Design review of the part built by this model. Coordinates are the model's own, in mm. A direction names the side the tool comes from. Coordinates: 2 decimals unless noted, no trailing zeros. Order: outer loops, then holes, each group sorted by start corner. A loop starts at its lowest first (then second) coordinate and runs counter-clockwise, first axis right, second up. Notation, with made-up numbers: M -34,6.25 L 15,6.25 A9 ccw 15,13.25 Z; hole C 17,-21 d9. An arc over 180 degrees is marked long. Answer in a Markdown table with one row per item.
Autodesk Inventor part; units mm, degrees
ref_plane "YZ Plane" through (0, 0, 0) normal (1, 0, 0) x (0, 1, 0)
ref_plane "XZ Plane" through (0, 0, 0) normal (0, 1, 0) x (-1, 0, 0)
ref_plane "XY Plane" through (0, 0, 0) normal (0, 0, 1) x (1, 0, 0)
sketch "スケッチ1" plane through (0, 0, 0) normal (0, 0, 1) x (1, 0, 0)
  line L0 (0, 0) -> (24.7487, 24.7487) construction
  line L1 (0, 0) -> (8.6903, 0) construction
  circle A0 centre (7.0711, 7.0711) radius 1.75
  circle A1 centre (12.0208, 12.0208) radius 1.75
  circle A2 centre (24.7487, 24.7487) radius 4.6188 construction
  circle A3 centre (24.7487, 24.7487) radius 8.6188
  line L2 (21.4828, 21.4828) -> (28.0147, 28.0147) construction
  circle A4 centre (29.2102, 23.5533) radius 4 construction
  circle A5 centre (21.4828, 21.4828) radius 4 construction
  circle A6 centre (23.5533, 29.2102) radius 4 construction
  circle A7 centre (29.2102, 23.5533) radius 1.5
  circle A8 centre (21.4828, 21.4828) radius 1.5
  circle A9 centre (23.5533, 29.2102) radius 1.5
  circle A10 centre (24.7487, 24.7487) radius 0.8755 construction
  circle A11 centre (0, 0) radius 5 construction
  arc A12 (5.7301, 8.1955) -> (7.0711, 7.0711) centre (0, 0) ccw
  arc A13 (-3.7643, 9.2644) -> (17.0249, 28.5731) centre (-18.8216, 46.3222) ccw
  arc A14 (28.5731, 17.0249) -> (9.2644, -3.7643) centre (46.3222, -18.8216) ccw
  line L3 (-4.8296, -1.2941) -> (-3.5355, 3.5355) construction
  line L4 (-3.5355, 3.5355) -> (1.2941, 4.8296) construction
  line L5 (1.2941, 4.8296) -> (4.8296, 1.2941) construction
  line L6 (4.8296, 1.2941) -> (3.5355, -3.5355) construction
  line L7 (3.5355, -3.5355) -> (-1.2941, -4.8296) construction
  line L8 (-1.2941, -4.8296) -> (-4.8296, -1.2941) construction
  arc A15 (-2.5213, 3.8073) -> (-3.8073, 2.5213) centre (-2.7931, 2.7931) ccw
  arc A16 (-4.5579, -0.2799) -> (-4.0872, -2.0366) centre (-3.8154, -1.0223) ccw
  arc A17 (-2.0366, -4.0872) -> (-0.2799, -4.5579) centre (-1.0223, -3.8154) ccw
  arc A18 (2.5213, -3.8073) -> (3.8073, -2.5213) centre (2.7931, -2.7931) ccw
  arc A19 (4.5579, 0.2799) -> (4.0872, 2.0366) centre (3.8154, 1.0223) ccw
  arc A20 (2.0366, 4.0872) -> (0.2799, 4.5579) centre (1.0223, 3.8154) ccw
  arc A21 (-2.5213, 3.8073) -> (0.2799, 4.5579) centre (-1.7707, 6.6085) ccw
  arc A22 (-4.5579, -0.2799) -> (-3.8073, 2.5213) centre (-6.6085, 1.7707) ccw
  arc A23 (-2.0366, -4.0872) -> (-4.0872, -2.0366) centre (-4.8377, -4.8377) ccw
  arc A24 (2.5213, -3.8073) -> (-0.2799, -4.5579) centre (1.7707, -6.6085) ccw
  arc A25 (4.5579, 0.2799) -> (3.8073, -2.5213) centre (6.6085, -1.7707) ccw
  arc A26 (2.0366, 4.0872) -> (4.0872, 2.0366) centre (4.8377, 4.8377) ccw
  circle A27 centre (0, 0) radius 6.05
  circle A28 centre (24.7487, 24.7487) radius 4 construction
  circle A29 centre (24.7487, 24.7487) radius 8
  line L9 (21.0131, 23.3188) -> (28.4844, 26.1787) construction
  circle A30 centre (21.9203, 27.5772) radius 4 construction
  circle A31 centre (27.5772, 21.9203) radius 4 construction
  circle A32 centre (21.9203, 27.5772) radius 3
  circle A33 centre (27.5772, 21.9203) radius 3
  line L10 (21.9203, 27.5772) -> (27.5772, 21.9203) construction
  circle A34 centre (21.9203, 27.5772) radius 1.75
  circle A35 centre (27.5772, 21.9203) radius 1.75
  point P0 (220.0202, -53)
  point P1 (-4.8296, -1.2941)
  point P2 (-1.2941, -4.8296)
  point P3 (3.5355, -3.5355)
  point P4 (4.8296, 1.2941)
  point P5 (4.0872, 2.0366)
  point P6 (4.5579, 0.2799)
  point P7 (3.8073, -2.5213)
  point P8 (2.5213, -3.8073)
  point P9 (-0.2799, -4.5579)
  point P10 (-2.0366, -4.0872)
  point P11 (-4.0872, -2.0366)
  point P12 (-4.5579, -0.2799)
  dimension "d2" = 3.5
  dimension "d15" = 10
  dimension "d0" = 35
  dimension "d1" = 45
  dimension "d3" = 3.5
  dimension "d4" = 10
  dimension "d5" = 7
  dimension "d10" = 17.2376
  dimension "d11" = 8
  dimension "d13" = 3
  dimension "d16" = 20
  dimension "d17" = 40
  dimension "d22" = 360
  dimension "d26" = 360
  dimension "d28" = 1.05
  dimension "d29" = 12.1
  dimension "d32" = 16
  dimension "d33" = 8
  dimension "d34" = 6
  dimension "d35" = 6
  dimension "d36" = 3.5
  dimension "d37" = 3.5
extrude "押し出し1" add sketch "スケッチ1" along normal blind 3 contours A0 A12 A13 A3 A14 | A0 A12 | A3 | A7 A33 | A33 A7 A35 | A7 A35 A33 | A8 | A9 A32 | A32 A9 A34 | A9 A34 A32 | A27 | A29
sketch "スケッチ2" plane through (0, 0, 3) normal (0, 0, 1) x (1, 0, 0)
  circle A0 centre (0, 0) radius 6.05
extrude "押し出し2" cut sketch "スケッチ2" against normal blind 1
equation "\"d37\" = d36"
properties part number "原動節" material "アルミニウム 2014-T4"
(1) Insertion check: pin 1 Ø1.5 at (x, z) = (1.5, 2.5) entering from -Y; pin 2 Ø1 at (y, z) = (13.5, 2) entering from +X. Each pin has a flat end and moves straight along its axis. Give the tip position at first contact, or say it passes through.
Return value:
| item | result |
|---|---|
| pin 1 | stops at y = -9.97 |
| pin 2 | stops at x = 23.46 |
(2) Draft analysis for pull direction X (two halves, no side actions). For faces 1 (the cylindrical face through (-6.873, -7.264, 1.479)), 2 (the cylindrical face through (8.548, 17.152, 1.479)), 3 (the flat face through (10, 10, 0)), 4 (the cylindrical face through (4.825, 1.309, 0.986)), state which applies: pulls with the +X half, pulls with the -X half, needs draft (parallel to the pull), parting line crosses it, or undercut.
Return value:
| item | result |
|---|---|
| face 1 | parting line crosses it |
| face 2 | pulls with the -X half |
| face 3 | needs draft |
| face 4 | undercut |
(3) Add section B-B, the plane z = 2.45. Give the boundary of the cut face in (x, y), and give its area (3 significant figures).
Return value:
| item | result |
|---|---|
| outline | M -3.76,9.26 A10 ccw long 9.26,-3.76 A40 cw 28.57,17.02 A8.62 ccw long 17.02,28.57 A40 cw Z; hole C 0,0 d12.1; hole C 7.07,7.07 d3.5; hole C 12.02,12.02 d3.5; hole C 21.92,27.58 d3.5; hole C 27.58,21.92 d3.5 |
| area | 636 mm2 |
(4) Add section A-A, the plane y = 13. Give the boundary of the cut face in (x, z).
Return value:
| item | result |
|---|---|
| outline | M 3.31,0 L 10.57,0 L 10.57,3 L 3.31,3 Z; M 13.47,0 L 22.09,0 L 22.09,3 L 13.47,3 Z |
(5) For line 1 along Y through (x, z) = (23, 0.6); line 2 along X through (y, z) = (22.5, 1.1); line 3 along X through (y, z) = (6, 1.85), list the stretches that pass through material, from the lowest coordinate up. Write a range as from..to.
Return value:
| item | result |
|---|---|
| line 1 | y = 13.68..26.2, 28.95..33.19 |
| line 2 | x = 13.31..25.93, 29.23..33.07 |
| line 3 | x = -8..5.69, 8.46..14.96 |
(6) Add section D-D, the plane x = 15.5. Give the boundary of the cut face in (y, z), and give its area (3 significant figures).
Return value:
| item | result |
|---|---|
| outline | M 6.67,0 L 25.78,0 L 25.78,3 L 6.67,3 Z |
| area | 57.3 mm2 |
(7) Add section C-C, the plane y = 23. Give the boundary of the cut face in (x, z).
Return value:
| item | result |
|---|---|
| outline | M 13.68,0 L 26.2,0 L 26.2,3 L 13.68,3 Z; M 28.95,0 L 33.19,0 L 33.19,3 L 28.95,3 Z |
(8) For faces 5 (the flat face through (13, 15, 3)), 6 (the cylindrical face through (-2.802, -2.772, 0.986)), list the 3-axis set-ups (+Z, -Z, +X, -X, +Y, -Y) from which the entire face can be reached by the end or side of a thin tool; tool diameter is ignored.
Return value:
| item | result |
|---|---|
| face 5 | +Z, +X, -X, +Y, -Y |
| face 6 | +Z, -Z |
